from build123d import *

# Parameters (mm, degrees)
BOSS_EXTRUDE3_DEPTH = 3
FILLET2_R           = 3
SKETCH6_R           = 4
BOSS_EXTRUDE4_DEPTH = 3
SKETCH7_R           = 2
CUT_EXTRUDE4_DEPTH  = 7


with BuildPart() as part:
    # Sketch5 → Boss-Extrude3 (new body)
    with BuildSketch(Plane(origin=(0, 0, 0), x_dir=(1, 0, 0), z_dir=(0, 1, 0))):
        with BuildLine():
            Line((-27.555542502, 26.418593403), (-5.236386006, 0))
            Line((-5.236386006, 0), (0, 6.198171191))
            Line((0, 6.198171191), (-21.444457498, 31.581406597))
            ThreePointArc((-21.444457498, 31.581406597), (-27.081406597, 32.055542502), (-27.555542502, 26.418593403))
        make_face()
        with BuildLine():
            Line((5.236386006, 0), (0, -6.198171191))
            Line((0, -6.198171191), (21.444457498, -31.581406597))
            ThreePointArc((21.444457498, -31.581406597), (27.081406597, -32.055542502), (27.555542502, -26.418593403))
            Line((27.555542502, -26.418593403), (5.236386006, 0))
        make_face()
        with BuildLine():
            Line((21.444457498, 31.581406597), (0, 6.198171191))
            Line((0, 6.198171191), (5.236386006, 0))
            Line((5.236386006, 0), (27.555542502, 26.418593403))
            ThreePointArc((27.555542502, 26.418593403), (27.081406597, 32.055542502), (21.444457498, 31.581406597))
        make_face()
        with BuildLine():
            Line((-5.236386006, 0), (-27.555542502, -26.418593403))
            ThreePointArc((-27.555542502, -26.418593403), (-27.081406597, -32.055542502), (-21.444457498, -31.581406597))
            Line((-21.444457498, -31.581406597), (0, -6.198171191))
            Line((0, -6.198171191), (-5.236386006, 0))
        make_face()
        Polygon((0, 6.198171191), (-5.236386006, 0), (0, -6.198171191), (5.236386006, 0), align=None)
    extrude(amount=BOSS_EXTRUDE3_DEPTH)

    # Fillet2
    fillet2_edges = [part.edges().sort_by_distance(p)[0] for p in [
        (0, 1.5, -6.198171191),
        (5.236386006, 1.5, 0),
        (0, 1.5, 6.198171191),
        (-5.236386006, 1.5, 0),
    ]]
    fillet(fillet2_edges, radius=FILLET2_R)

    # Sketch6 → Boss-Extrude4 (add)
    with BuildSketch(Plane(origin=(0, 3, 0), x_dir=(1, 0, 0), z_dir=(0, 1, 0))):
        with Locations((-24.5, 29)):
            Circle(SKETCH6_R)
        with Locations((24.5, 29)):
            Circle(SKETCH6_R)
        with Locations((-24.5, -29)):
            Circle(SKETCH6_R)
        with Locations((24.5, -29)):
            Circle(SKETCH6_R)
    extrude(amount=BOSS_EXTRUDE4_DEPTH)

    # Sketch7 → Cut-Extrude4 (cut, through all)
    with BuildSketch(Plane(origin=(0, 6, 0), x_dir=(1, 0, 0), z_dir=(0, 1, 0))):
        with Locations((-24.5, -29)):
            Circle(SKETCH7_R)
        with Locations((-24.5, 29)):
            Circle(SKETCH7_R)
        with Locations((24.5, 29)):
            Circle(SKETCH7_R)
        with Locations((24.5, -29)):
            Circle(SKETCH7_R)
    extrude(amount=-CUT_EXTRUDE4_DEPTH, mode=Mode.SUBTRACT)


solid = part.part
Design review of the part built by this model. Coordinates are the model's own, in mm. A direction names the side the tool comes from. Coordinates: 2 decimals unless noted, no trailing zeros. Loops run counter-clockwise (first coordinate to the right, second up) from the corner with the lowest first, then second, coordinate; pieces in that order, holes last.
Item 1: Add section D-D (x = -24.5). Write out the cut boundary in (y, z), and give its area (3 significant figures).
Completed:
outline: (0, -33) - (6, -33) - (6, -31) - (0, -31) - close; (0, -27) - (6, -27) - (6, -25) - (3, -25) - (3, -22.8) - (0, -22.8) - close; (0, 22.8) - (3, 22.8) - (3, 25) - (6, 25) - (6, 27) - (0, 27) - close; (0, 31) - (6, 31) - (6, 33) - (0, 33) - close
area: 61.2 mm2
Item 2: Clearance check with flat-ended pins moving along their axes: pin 1 (2.5 mm diameter, centred on x = 24.5, z = -29, fed in from -Y); pin 2 (3 mm diameter, centred on y = 1, z = -19, fed in from -X); pin 3 (3 mm diameter, centred on y = 3, z = 7.5, fed in from +X); pin 4 (2 mm diameter, centred on x = -20.5, y = 0.5, fed in from +Z). State where each tip first meets the part, or that it passes through.
Completed:
pin 1: passes through
pin 2: stops at x = -22.56
pin 3: stops at x = 12.84
pin 4: stops at z = 31.65
Item 3: Add section B-B (z = 16). Write out the cut boundary in (x, y).
Completed:
outline: (-18.75, 0) - (-8.28, 0) - (-8.28, 3) - (-18.75, 3) - close; (8.28, 0) - (18.75, 0) - (18.75, 3) - (8.28, 3) - close
Item 4: For faces 1 (the flat face through (-17.36, 1.48, -14.35)), 2 (the cylindrical face through (-27.7, 3.6, 31.4)), 3 (the flat face through (17.36, 1.48, 14.35)), list the 3-axis set-ups (+Z, -Z, +X, -X, +Y, -Y) from which the entire face can be reached by the end or side of a thin tool; tool diameter is ignored.
Completed:
face 1: -X, +Y, -Y
face 2: +Y
face 3: +X, +Y, -Y
Item 5: Add section C-C (x = 12.5). Write out the cut boundary in (y, z).
Completed:
outline: (0, -20.99) - (3, -20.99) - (3, -8.6) - (0, -8.6) - close; (0, 8.6) - (3, 8.6) - (3, 20.99) - (0, 20.99) - close
Item 6: Add section A-A (y = 4.8). Write out the cut boundary in (x, z).
Completed:
outline: circle Ø8 at (-24.5, -29); circle Ø8 at (-24.5, 29); circle Ø8 at (24.5, -29); circle Ø8 at (24.5, 29); hole circle Ø4 at (-24.5, -29); hole circle Ø4 at (-24.5, 29); hole circle Ø4 at (24.5, -29); hole circle Ø4 at (24.5, 29)
Item 7: Wall thickness on L1, parallel to X at y = 4.75, z = -29; L2, parallel to Z at x = -24.5, y = 4.05; L3, parallel to X at y = 2.8, z = 29: over which ranges is each line inside the solid? List them lowest first.
Completed:
L1: x = -28.5 to -26.5, -22.5 to -20.5, 20.5 to 22.5, 26.5 to 28.5
L2: z = -33 to -31, -27 to -25, 25 to 27, 31 to 33
L3: x = -28.5 to -26.5, -22.5 to -19.26, 19.26 to 22.5, 26.5 to 28.5
